Design review of the part built by this model. Coordinates are the model's own, in mm. A direction names the side the tool comes from. Round coordinates to 2 decimals unless told otherwise and drop trailing zeros. Order: outer loops, then holes, each group sorted by start corner. A loop starts at its lowest first (then second) coordinate and runs counter-clockwise, first axis right, second up. Notation, with made-up numbers: M 57.25,66 L 93.25,66 A6 cw 93.25,70 Z; hole C -31,52.5 d8. An arc over 180 degrees is marked long. Use a Markdown table: item, result. Add a question column.
(1) The part is to be moulded in two halves that separate along X. For faces 6 (the face through (0, 134, 39)), 7 (the face through (10, 70, 41)), 8 (the face through (3, 56, 80)), say which applies: released by +X, released by -X, zero draft, split by the parting line, or undercut.
(2) Take a section at D-D (x = -20.5). Write out the cut boundary in (y, z), then the cut area to 3 significant figures.
(3) Take a section at A-A (y = 40.5). Write out the cut boundary in (x, z).
(4) Take a section at C-C (y = 148). Write out the cut boundary in (x, z), then the cut area to 3 significant figures.
(5) Machinability: for faces 1 (the face through (10.335, 354.569, 77.834)), 2 (the face through (5, 42, 41)), 3 (the face through (10.14, 114.591, 67.675)), 4 (the face through (3, 56, 0)), 5 (the face through (10.14, 115.221, 12.675)), which of the approach directions +Z, -Z, +X, -X, +Y, -Y give a long, thin tool a straight path to every point of the face, cutting with its end or side? Answer none if there is none.
(6) For pin 1 (3 mm diameter, centred on y = 53.06, z = 70, fed in from +X); pin 2 (6.5 mm diameter, centred on y = 195, z = 32.5, fed in from -X); pin 3 (1 mm diameter, centred on x = -19.5, z = 47.5, fed in from -Y); pin 4 (5 mm diameter, centred on x = 10.5, y = 132, fed in from -Z), all flat-tipped, find the tip position at first contact; note any pin that passes through.
(7) Take a section at B-B (z = 19). Write out the cut boundary in (x, y), then the cut area to 3 significant figures.
(8) To check wall thickness, follow probe 1 along Z at (x, y) = (11, 175); probe 2 along Y at (x, z) = (16.25, 32.5); probe 3 along X at (y, z) = (43.5, 20). State the ranges of each line that lie inside material, in increasing order. Write a range as from..to.
```python
from build123d import *

# Parameters (mm, degrees)
SUPPORT_BALISE_W                           = 20
SUPPORT_BALISE_H                           = 350
SUPPORT_BALISE_BOSSAGE_DEPTH               = 80
ESQUISSE3_W                                = 80
ESQUISSE3_H                                = 80
SUPPORT_CHEVAL_ENLEVEMENT_DE_MATIERE_DEPTH = 10
ESQUISSE8_W                                = 10
ESQUISSE8_H                                = 70
SUPPORT_CHEVAL_DEPTH                       = 80
VIS_REACH                                  = 376.466
SERRAGE_VIS_R                              = 2.5
VIS_DIRECTION_2_DEPTH                      = 375.466286867
ENL_V_MAT_EXTRU_5_DEPTH                    = 20
POUR_IMPRESSION_R                          = 15
FIXATION_POUR_ASSEMBLAGE_R                 = 2
VIS_POUR_ASSEMBLAGE_DEPTH                  = 20


with BuildPart() as part:
    # Support Balise → Support balise bossage (new body)
    with BuildSketch(Plane.XY):
        with Locations((10, 175)):
            Rectangle(SUPPORT_BALISE_W, SUPPORT_BALISE_H)
    extrude(amount=SUPPORT_BALISE_BOSSAGE_DEPTH)

    # Esquisse3 → Support Cheval enlevement de matiere (add)
    with BuildSketch(Plane(origin=(0, 350, 0), x_dir=(1, 0, 0), z_dir=(0, 1, 0))):
        with Locations((-20, -40)):
            Rectangle(ESQUISSE3_W, ESQUISSE3_H)
    extrude(amount=SUPPORT_CHEVAL_ENLEVEMENT_DE_MATIERE_DEPTH)

    # Esquisse8 → Support Cheval (cut)
    with BuildSketch(Plane.XY.offset(80)):
        with Locations((10, 35)):
            Rectangle(ESQUISSE8_W, ESQUISSE8_H)
    extrude(amount=-SUPPORT_CHEVAL_DEPTH, mode=Mode.SUBTRACT)

    # Vis: up to this face of the body (flat: up to its plane)
    vis_end = Plane(part.part.faces().sort_by_distance((0, 175, 40))[0])
    # Serrage vis → Vis (cut, up to the picked face)
    with BuildSketch(Plane(origin=(5, 0, 0), x_dir=(0, 0, -1), z_dir=(1, 0, 0)), mode=Mode.PRIVATE) as vis_sk1:
        with Locations((-70, 11.284552026)):
            Circle(SERRAGE_VIS_R)
    vis_tool1 = split(extrude(vis_sk1.sketch, amount=-VIS_REACH, mode=Mode.PRIVATE), bisect_by=vis_end, keep=Keep.BOTH, mode=Mode.PRIVATE)
    # Serrage vis → Vis (cut, up to the picked face)
    with BuildSketch(Plane(origin=(5, 0, 0), x_dir=(0, 0, -1), z_dir=(1, 0, 0)), mode=Mode.PRIVATE) as vis_sk2:
        with Locations((-70, 53.057184379)):
            Circle(SERRAGE_VIS_R)
    vis_tool2 = split(extrude(vis_sk2.sketch, amount=-VIS_REACH, mode=Mode.PRIVATE), bisect_by=vis_end, keep=Keep.BOTH, mode=Mode.PRIVATE)
    # Serrage vis → Vis (cut, up to the picked face)
    with BuildSketch(Plane(origin=(5, 0, 0), x_dir=(0, 0, -1), z_dir=(1, 0, 0)), mode=Mode.PRIVATE) as vis_sk3:
        with Locations((-10, 53.057184379)):
            Circle(SERRAGE_VIS_R)
    vis_tool3 = split(extrude(vis_sk3.sketch, amount=-VIS_REACH, mode=Mode.PRIVATE), bisect_by=vis_end, keep=Keep.BOTH, mode=Mode.PRIVATE)
    # Serrage vis → Vis (cut, up to the picked face)
    with BuildSketch(Plane(origin=(5, 0, 0), x_dir=(0, 0, -1), z_dir=(1, 0, 0)), mode=Mode.PRIVATE) as vis_sk4:
        with Locations((-10, 11.284552026)):
            Circle(SERRAGE_VIS_R)
    vis_tool4 = split(extrude(vis_sk4.sketch, amount=-VIS_REACH, mode=Mode.PRIVATE), bisect_by=vis_end, keep=Keep.BOTH, mode=Mode.PRIVATE)
    # Serrage vis → Vis (cut, up to the picked face)
    with BuildSketch(Plane(origin=(5, 0, 0), x_dir=(0, 0, -1), z_dir=(1, 0, 0)), mode=Mode.PRIVATE) as vis_sk5:
        with Locations((-40, 32.170868202)):
            Circle(SERRAGE_VIS_R)
    vis_tool5 = split(extrude(vis_sk5.sketch, amount=-VIS_REACH, mode=Mode.PRIVATE), bisect_by=vis_end, keep=Keep.BOTH, mode=Mode.PRIVATE)
    add(vis_tool1.solids().sort_by(Axis((5, 11.284552, 70), (-1, 0, 0)))[0], mode=Mode.SUBTRACT)
    add(vis_tool2.solids().sort_by(Axis((5, 53.057184, 70), (-1, 0, 0)))[0], mode=Mode.SUBTRACT)
    add(vis_tool3.solids().sort_by(Axis((5, 53.057184, 10), (-1, 0, 0)))[0], mode=Mode.SUBTRACT)
    add(vis_tool4.solids().sort_by(Axis((5, 11.284552, 10), (-1, 0, 0)))[0], mode=Mode.SUBTRACT)
    add(vis_tool5.solids().sort_by(Axis((5, 32.170868, 40), (-1, 0, 0)))[0], mode=Mode.SUBTRACT)

    # Serrage vis → Vis direction 2 (cut)
    with BuildSketch(Plane(origin=(5, 0, 0), x_dir=(0, 0, -1), z_dir=(1, 0, 0))):
        with Locations((-70, 11.284552026)):
            Circle(SERRAGE_VIS_R)
        with Locations((-70, 53.057184379)):
            Circle(SERRAGE_VIS_R)
        with Locations((-10, 53.057184379)):
            Circle(SERRAGE_VIS_R)
        with Locations((-10, 11.284552026)):
            Circle(SERRAGE_VIS_R)
        with Locations((-40, 32.170868202)):
            Circle(SERRAGE_VIS_R)
    extrude(amount=VIS_DIRECTION_2_DEPTH, mode=Mode.SUBTRACT)

    # Design → Enlèv. mat.-Extru.5 (cut)
    with BuildSketch(Plane(origin=(20, 0, 0), x_dir=(0, 0, -1), z_dir=(1, 0, 0))):
        Polygon((-55, 315), (-80, 360), (-80, 92.406088827), (-55, 137.406088827), align=None)
        Polygon((0, 92.406088827), (0, 360), (-25, 315), (-25, 137.406088827), align=None)
    extrude(amount=-ENL_V_MAT_EXTRU_5_DEPTH, mode=Mode.SUBTRACT)

    # Pour Impression
    # the kernel refuses this fillet: 15 mm, written as the material it adds along each edge
    with BuildSketch(Plane(origin=(0, 392.780897855, -18.211609919), x_dir=(1, 0, 0), z_dir=(0, -0.8741572761215375, 0.48564293117863266))) as pour_impression_piece_1_section:
        with BuildLine():
            CenterArc((POUR_IMPRESSION_R, -POUR_IMPRESSION_R), POUR_IMPRESSION_R, 90, 90)
            Line((0, -POUR_IMPRESSION_R), (0, 0))
            Line((0, 0), (POUR_IMPRESSION_R, 0))
        make_face()
    pour_impression_piece_1 = extrude(amount=86.439589046, mode=Mode.PRIVATE)
    pour_impression_piece_1 = split(pour_impression_piece_1, bisect_by=Plane(origin=(4.741525676, 350, 2.029382941), z_dir=(0, 1, 0)), keep=Keep.TOP, mode=Mode.PRIVATE)
    pour_impression_piece_1 = split(pour_impression_piece_1, bisect_by=Plane(origin=(4.741525676, 353.652889294, 0), z_dir=(0, 0, 1)), keep=Keep.TOP, mode=Mode.PRIVATE)
    add(pour_impression_piece_1)
    with BuildSketch(Plane(origin=(0, 317.219102145, 56.232834525), x_dir=(1, 0, 0), z_dir=(0, 0.8741572761215377, 0.4856429311786322))) as pour_impression_piece_2_section:
        with BuildLine():
            CenterArc((POUR_IMPRESSION_R, -POUR_IMPRESSION_R), POUR_IMPRESSION_R, 90, 90)
            Line((0, -POUR_IMPRESSION_R), (0, 0))
            Line((0, 0), (POUR_IMPRESSION_R, 0))
        make_face()
    pour_impression_piece_2 = extrude(amount=86.439589046, mode=Mode.PRIVATE)
    pour_impression_piece_2 = split(pour_impression_piece_2, bisect_by=Plane(origin=(4.741525676, 350, 77.970617059), z_dir=(0, 1, 0)), keep=Keep.TOP, mode=Mode.PRIVATE)
    pour_impression_piece_2 = split(pour_impression_piece_2, bisect_by=Plane(origin=(4.741525676, 353.652889294, 80), z_dir=(0, 0, -1)), keep=Keep.TOP, mode=Mode.PRIVATE)
    add(pour_impression_piece_2)

    # Fixation pour assemblage → Vis pour Assemblage (cut)
    with BuildSketch(Plane(origin=(20, 0, 0), x_dir=(0, 0, -1), z_dir=(1, 0, 0))):
        with Locations((-47.5, 195)):
            Circle(FIXATION_POUR_ASSEMBLAGE_R)
        with Locations((-32.5, 195)):
            Circle(FIXATION_POUR_ASSEMBLAGE_R)
        with Locations((-32.5, 175)):
            Circle(FIXATION_POUR_ASSEMBLAGE_R)
        with Locations((-47.5, 175)):
            Circle(FIXATION_POUR_ASSEMBLAGE_R)
    extrude(amount=-VIS_POUR_ASSEMBLAGE_DEPTH, mode=Mode.SUBTRACT)


solid = part.part
```
Verdict:
| question | item | result |
|---|---|---|
| 1 | face 6 | released by -X |
| 1 | face 7 | undercut |
| 1 | face 8 | zero draft |
| 2 | outline | M 350,0 L 360,0 L 360,80 L 350,80 Z |
| 2 | area | 800 mm^2 |
| 3 | outline | M 0,0 L 5,0 L 5,80 L 0,80 Z; M 15,0 L 20,0 L 20,80 L 15,80 Z |
| 4 | outline | M 0,25 L 20,25 L 20,55 L 0,55 Z |
| 4 | area | 600 mm^2 |
| 5 | face 1 | +Z, +X |
| 5 | face 2 | +Z, -Z, -Y |
| 5 | face 3 | +Z, +X, -X |
| 5 | face 4 | -Z, +X, -X, +Y, -Y |
| 5 | face 5 | -Z, +X, -X |
| 6 | pin 1 | passes through |
| 6 | pin 2 | stops at x = 0 |
| 6 | pin 3 | stops at y = 350 |
| 6 | pin 4 | stops at z = 20.61 |
| 7 | outline | M -60,350 L 0,350 L 0,325.8 L 20,325.8 L 20,360 L -60,360 Z; M 0,0 L 5,0 L 5,70 L 15,70 L 15,0 L 20,0 L 20,126.61 L 0,126.61 Z |
| 7 | area | 3,120 mm^2 |
| 8 | probe 1 | z = 25..30.5, 34.5..45.5, 49.5..55 |
| 8 | probe 2 | y = 0..173, 177..193, 197..360 |
| 8 | probe 3 | x = 0..5, 15..20 |
